Geometry check sheet. Reference: the model listing, model coordinates, mm. A direction names the side the tool comes from. Give positions to 0.01 mm unless a question says otherwise; leave off trailing zeros. Order: outer loops, then holes, each group sorted by start corner. A loop starts at its lowest first (then second) coordinate and runs counter-clockwise, first axis right, second up. Notation, with made-up numbers: M -28.75,19.25 L 10.25,19.25 A16 cw 10.25,28.25 Z; hole C 44,86.25 d1. An arc over 180 degrees is marked long. Answer as CSV lines item,"result". Start each with the question number.
Q1. Section check B-B, the plane y = -3. Record the boundary of the cut face in (x, z) (1 decimal), then the cut area to 3 significant figures.
Q2. Mould release check, pull along Z, two halves, no side actions. Record for faces 4 (the flat face through (3, 0, -5)), 5 (the flat face through (-3.8, 1.6, 0.19)): +Z half, -Z half, draft (parallel to the pull), parting line (faces both ways), or undercut.
Q3. Thickness scan on line 1 (Z direction, x = 0, y = 0.25); line 2 (X direction, y = 0.25, z = 0); line 3 (X direction, y = 1.6, z = 0) (3 decimals). Record the ranges inside material, lowest first.
Q4. Section check A-A, the plane z = 12. Record the boundary of the cut face in (x, y), then the cut area to 3 significant figures.
Q5. Go/stop test with flat-tipped pins: pin 1 (2 mm diameter, centred on x = -2.5, y = 0.5, fed in from -Z); pin 2 (1 mm diameter, centred on x = 2, z = 0, fed in from +Y); pin 3 (4 mm diameter, centred on x = 1.5, z = -10, fed in from +Y). Record where each tip stops, or that it passes through.
Q6. Set-up check for faces 1 (the cylindrical face through (2.833, -2.12, 0.372)), 2 (the flat face through (0.191, 1.6, -3.8)), 3 (the flat face through (-8.116, 0.952, -8.226)): record each of +Z, -Z, +X, -X, +Y, -Y from which the full face is reachable in a straight line by a thin tool's end or side.
Q7. Section check C-C, the plane y = -1.25. Record the boundary of the cut face in (x, z) (1 decimal).
```python
from build123d import *

# Parameters (mm, degrees)
EXTRUDE4_DEPTH          = 1.9304
SKETCH2_R               = 0.6604
CUT_EXTRUDE1_DEPTH      = 19.722050478
CIRPATTERN4_COUNT       = 6
CUT_EXTRUDE2_DEPTH      = 12.7
CUT_EXTRUDE2_DEPTH_BACK = 12.7
SKETCH3_R               = 1.397
SKETCH4_R               = 4.445
CUT_EXTRUDE3_DEPTH      = 0.635
SKETCH5_R               = 3.4925
SKETCH5_R_2             = 3.175
EXTRUDE5_DEPTH          = 1.143
RIB10_REACH             = 26.438
SKETCH8_WALL_W          = 52.220152264
SKETCH8_WALL_H          = 0.381
CIRPATTERN5_COUNT       = 8
SKETCH10_R              = 5.08
EXTRUDE6_DEPTH          = 0.762
FILLET2_R               = 0.508
SKETCH11_R              = 4.064
EXTRUDE7_DEPTH          = 3.048
FILLET3_R               = 0.889
SKETCH12_R              = 2.8575
CUT_EXTRUDE5_DEPTH      = 3.429
SKETCH14_R              = 1.397
CUT_EXTRUDE6_DEPTH      = 25.557003564
SKETCH15_R              = 0.3175
CUT_EXTRUDE7_DEPTH      = 25.984806887
CIRPATTERN7_COUNT       = 6


with BuildPart() as part:
    # Sketch1 → Extrude4 (new body)
    with BuildSketch(Plane(origin=(0, 0, 0), x_dir=(1, 0, 0), z_dir=(0, 1, 0))):
        with BuildLine():
            Line((5.775220615, -3.829827046), (0, 0))
            Line((0, 0), (5.775220615, 3.829827046))
            Line((5.775220615, 3.829827046), (6.35029977, 3.829827046))
            Line((6.35029977, 3.829827046), (6.35029977, 3.494998084))
            Line((6.35029977, 3.494998084), (15.87469147, 2.35207108))
            ThreePointArc((15.87469147, 2.35207108), (18.22419147, 0.00257108), (15.87469147, -2.34692892))
            Line((15.87469147, -2.34692892), (6.34969147, -3.48992892))
            Line((6.34969147, -3.48992892), (6.34969147, -3.829827046))
            Line((6.34969147, -3.829827046), (5.775220615, -3.829827046))
        make_face()
    extrude4 = extrude(amount=EXTRUDE4_DEPTH)

    # Sketch2 → Cut-Extrude1 (cut, through all)
    with BuildSketch(Plane(origin=(0, 1.9304, 0), x_dir=(-1, 0, 0), z_dir=(0, 1, 0))):
        with Locations((-6.342552501, -4.149920748)):
            Circle(SKETCH2_R)
        with Locations((-6.342552501, 4.149920748)):
            Circle(SKETCH2_R)
    extrude(amount=-CUT_EXTRUDE1_DEPTH, mode=Mode.SUBTRACT)

    # CirPattern4: Extrude4 ×6 about axis
    cirpattern4_axis = Axis((0, 0, 0), (0, 1, 0))
    for i in range(1, CIRPATTERN4_COUNT):
        add(extrude4.rotate(cirpattern4_axis, i * 360 / CIRPATTERN4_COUNT))

    # Sketch3 → Cut-Extrude2 (cut, two sides: drawn at the far end of the back side and taken through both)
    with BuildSketch(Plane(origin=(0, 1.9304, 0), x_dir=(-1, 0, 0), z_dir=(0, 1, 0)).offset(-CUT_EXTRUDE2_DEPTH_BACK)):
        with Locations(Location((0, 0, 0), (0, 0, 90))):
            Circle(SKETCH3_R)
    extrude(amount=CUT_EXTRUDE2_DEPTH + CUT_EXTRUDE2_DEPTH_BACK, mode=Mode.SUBTRACT)

    # Sketch4 → Cut-Extrude3 (cut)
    with BuildSketch(Plane(origin=(0, 1.9304, 0), x_dir=(-1, 0, 0), z_dir=(0, 1, 0))):
        with Locations(Location((0, 0, 0), (0, 0, 90))):
            Circle(SKETCH4_R)
    extrude(amount=-CUT_EXTRUDE3_DEPTH, mode=Mode.SUBTRACT)

    # Sketch5 → Extrude5 (add)
    with BuildSketch(Plane(origin=(0, 1.2954, 0), x_dir=(-1, 0, 0), z_dir=(0, 1, 0))):
        with Locations(Location((0, 0, 0), (0, 0, 90))):
            Circle(SKETCH5_R)
        with Locations(Location((0, 0, 0), (0, 0, 90))):
            Circle(SKETCH5_R_2, mode=Mode.SUBTRACT)
    extrude(amount=EXTRUDE5_DEPTH)

    # Sketch8 wall → Rib10 (add, up to next)
    with BuildSketch(Plane(origin=(-3.967749561, 1.770078976, 0), x_dir=(-0.70753138537, -0.706681921883, 0), z_dir=(0.706681921883, -0.70753138537, 0)), mode=Mode.PRIVATE) as rib10_sk1:
        Rectangle(SKETCH8_WALL_W, SKETCH8_WALL_H)
    rib10_tool1 = extrude(rib10_sk1.sketch, amount=RIB10_REACH, mode=Mode.PRIVATE) - part.part
    rib10 = rib10_tool1.solids().sort_by_distance((-3.967749561, 1.770078976, 0))[0]
    add(rib10)

    # CirPattern5: Rib10 ×8 about axis
    cirpattern5_axis = Axis((0, 0, 0), (0, 1, 0))
    for i in range(1, CIRPATTERN5_COUNT):
        add(rib10.rotate(cirpattern5_axis, i * 360 / CIRPATTERN5_COUNT))

    # Sketch10 → Extrude6 (add)
    with BuildSketch(Plane.XZ):
        with Locations(Location((0, 0, 0), (0, 0, 90))):
            Circle(SKETCH10_R)
    extrude(amount=EXTRUDE6_DEPTH)

    # Fillet2
    fillet2_edges = [part.edges().sort_by_distance(p)[0] for p in [
        (0, 0, -5.08),
    ]]
    fillet(fillet2_edges, radius=FILLET2_R)

    # Sketch11 → Extrude7 (add)
    with BuildSketch(Plane.XZ.offset(0.762)):
        with Locations(Location((0, 0, 0), (0, 0, 90))):
            Circle(SKETCH11_R)
    extrude(amount=EXTRUDE7_DEPTH)

    # Fillet3
    fillet3_edges = [part.edges().sort_by_distance(p)[0] for p in [
        (0, -0.762, -4.064),
    ]]
    fillet(fillet3_edges, radius=FILLET3_R)

    # Sketch12 → Cut-Extrude5 (cut)
    with BuildSketch(Plane.XZ.offset(3.81)):
        with Locations(Location((0, 0, 0), (0, 0, 270))):
            Circle(SKETCH12_R)
    extrude(amount=-CUT_EXTRUDE5_DEPTH, mode=Mode.SUBTRACT)

    # Sketch14 → Cut-Extrude6 (cut, through all)
    with BuildSketch(Plane.XZ.offset(0.381)):
        with Locations(Location((0, 0, 0), (0, 0, 90))):
            Circle(SKETCH14_R)
    extrude(amount=-CUT_EXTRUDE6_DEPTH, mode=Mode.SUBTRACT)

    # Sketch15 → Cut-Extrude7 (cut, symmetric)
    with BuildSketch(Plane(origin=(0, 1.9304, 0), x_dir=(-1, 0, 0), z_dir=(0, 1, 0))):
        with Locations((-6.48724684, -3.751940905)):
            Circle(SKETCH15_R)
    cut_extrude7 = extrude(amount=CUT_EXTRUDE7_DEPTH, both=True, mode=Mode.SUBTRACT)

    # CirPattern7: Cut-Extrude7 ×6 about axis
    cirpattern7_axis = Axis((0, 0, 0), (0, 1, 0))
    for i in range(1, CIRPATTERN7_COUNT):
        add(cut_extrude7.rotate(cirpattern7_axis, i * 360 / CIRPATTERN7_COUNT), mode=Mode.SUBTRACT)


solid = part.part
```
Answer block:
1,outline,"C 0,0 d8.1; hole C 0,0 d5.7"
1,area,"26.2 mm2"
2,face 4,"draft"
2,face 5,"undercut"
3,line 1,"z = -7.18 to -1.4, 1.4 to 7.18"
3,line 2,"x = -18.22 to -1.4, 1.4 to 18.22"
3,line 3,"x = -18.224 to -4.445, -4.138 to -3.175, 3.175 to 4.138, 4.445 to 18.224"
4,outline,"M -9.72,0 L -3.71,0 L -3.71,1.93 L -9.72,1.93 Z; M 3.72,0 L 9.73,0 L 9.73,1.93 L 3.72,1.93 Z"
4,area,"23.2 mm2"
5,pin 1,"stops at z = -11.71"
5,pin 2,"stops at y = 1.3"
5,pin 3,"stops at y = 1.93"
6,face 1,"-Y"
6,face 2,"+Y"
6,face 3,"-X, +Y, -Y"
7,outline,"C 0,0 d8.3; hole C 0,0 d5.7"
